Job drawing, mm, ordinate dimensions from the low corner. One solid piece. A direction names the side the tool comes from. Round coordinates to 2 decimals unless told otherwise and drop trailing zeros. Write each loop counter-clockwise with the first axis right and the second up, starting at its lowest first coordinate (ties: lowest second). Pieces come first, ordered by that corner, then holes. Notation, with made-up numbers: M -14,-31 L 34,-31 A23 ccw 34,-21 Z; hole C -11,50 d4. An arc over 180 degrees is marked long. Write each question's results on one line, items separated by ' | '. Start each with the question number.
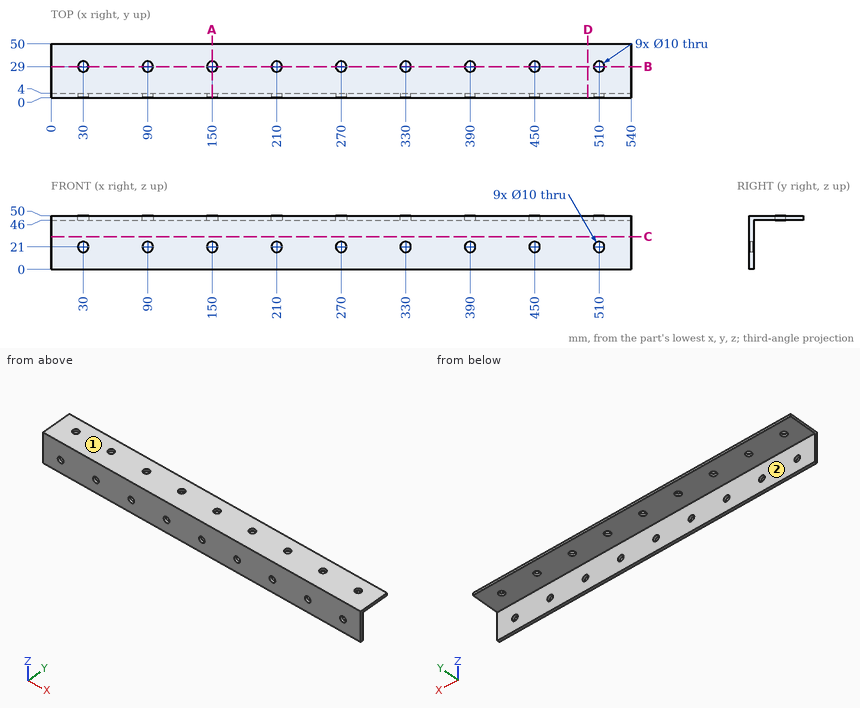
1) Saw through at D-D, the plane x = 499.5. Write the cut outline in (y, z), plus the area to 3 significant figures.
2) Wall check: line 1 along Y through (x, z) = (450, 47.05); line 2 along Z through (x, y) = (68, 14); line 3 along Y through (x, z) = (287.5, 29.5). Give the ranges that are in metal, low to high. Write a range as from..to.
3) Saw through at C-C, the plane z = 30.5. Write the cut outline in (x, y).
4) 3-axis set-ups, long thin cutter, end or side, ignore diameter. For the marked faces 1 and 2: which of +Z, -Z, +X, -X, +Y, -Y reach the whole face in a straight line?
5) Saw through at A-A, the plane x = 150. Write the cut outline in (y, z).
6) Drop flat-ended pins along their axis: pin 1 Ø8 at (x, y) = (450, 29) entering from +Z; pin 2 Ø1.5 at (x, z) = (143.5, 27) entering from +Y; pin 3 Ø14 at (x, y) = (309.5, 37) entering from -Z. Give the stop position or say it passes through.
7) Saw through at B-B, the plane y = 29. State how many separate pieces and enclosed holes the cut face has, plus the area to 3 significant figures.
Filled sheet:
1) outline: M 0,0 L 4,0 L 4,46 L 50,46 L 50,50 L 0,50 Z | area: 384 mm^2
2) line 1: y = 0..24, 34..50 | line 2: z = 46..50 | line 3: y = 0..4
3) outline: M 0,0 L 540,0 L 540,4 L 0,4 Z
4) face 1: +Z, +X, -X, +Y, -Y | face 2: -Z, +X, -X, +Y
5) outline: M 0,0 L 4,0 L 4,16 L 0,16 Z; M 0,26 L 4,26 L 4,46 L 24,46 L 24,50 L 0,50 Z; M 34,46 L 50,46 L 50,50 L 34,50 Z
6) pin 1: passes through | pin 2: stops at y = 4 | pin 3: stops at z = 46
7) separate pieces: 10 | enclosed holes: 0 | area: 1,800 mm^2
